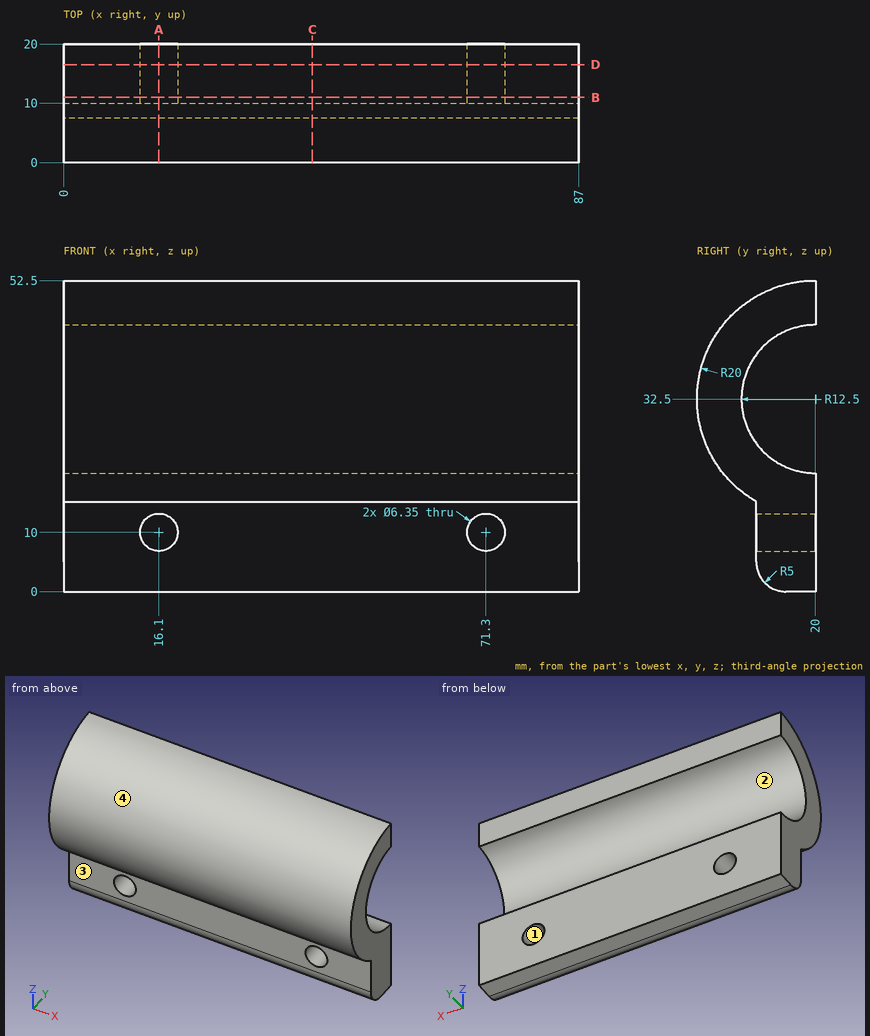
Here's the drawing with two shaded views (mm, measured from the low corner). I have some questions. Coordinates: 2 decimals unless noted, no trailing zeros. Loops run counter-clockwise (first coordinate to the right, second up) from the corner with the lowest first, then second, coordinate; pieces in that order, holes last. Notation, with made-up numbers: (24, 89.25) -> (69, 89.25) arc R24 ccw to (69, 111.25) -> close; hole circle Ø10 at (65.5, -38.5). An arc over 180 degrees is marked (long way). Answer in a Markdown table with one row per item.
(1) Imagine slicing it at A-A (x = 16.1). List the corners of the cut face in (y, z) for me (1 decimal), plus the area to 3 significant figures.
Results found:
| item | result |
|---|---|
| outline | (10, 5) arc R5 ccw to (15, 0) -> (20, 0) -> (20, 6.8) -> (10, 6.8) -> close; (10, 13.2) -> (20, 13.2) -> (20, 20) arc R12.5 cw to (20, 45) -> (20, 52.5) arc R20 ccw to (10, 15.2) -> close |
| area | 448 mm^2 |
(2) Imagine slicing it at B-B (y = 11). List the corners of the cut face in (x, z) for me (3 decimals), plus the area to 3 significant figures.
Results found:
| item | result |
|---|---|
| outline | (0, 2) -> (87, 2) -> (87, 23.825) -> (0, 23.825) -> close; (0, 41.175) -> (87, 41.175) -> (87, 50.361) -> (0, 50.361) -> close; hole circle Ø6.35 at (16.1, 10); hole circle Ø6.35 at (71.3, 10) |
| area | 2,630 mm^2 |
(3) Thinking about a two-plate mould opening in Z: for the marked faces 1, 2, 3 and 4, which applies, released by +Z, released by -Z, zero draft, split by the parting line, or undercut?
Results found:
| item | result |
|---|---|
| face 1 | undercut |
| face 2 | undercut |
| face 3 | zero draft |
| face 4 | split by the parting line |
(4) Will these pins go through, and if not, where does the flat tip stop? pin 1 Ø7.5 at (x, z) = (71.3, 10) entering from -Y; pin 2 Ø5.5 at (x, z) = (16.1, 10) entering from -Y; pin 3 Ø8 at (x, y) = (73, 6.5) entering from +Z; pin 4 Ø6 at (x, y) = (21, 14) entering from +Z.
Results found:
| item | result |
|---|---|
| pin 1 | stops at y = 10 |
| pin 2 | passes through |
| pin 3 | stops at z = 50.1 |
| pin 4 | stops at z = 52.27 |
(5) Imagine slicing it at D-D (y = 16.5). List the corners of the cut face in (x, z) for me (3 decimals), plus the area to 3 significant figures.
Results found:
| item | result |
|---|---|
| outline | (0, 0) -> (87, 0) -> (87, 20.5) -> (0, 20.5) -> close; (0, 44.5) -> (87, 44.5) -> (87, 52.191) -> (0, 52.191) -> close; hole circle Ø6.35 at (16.1, 10); hole circle Ø6.35 at (71.3, 10) |
| area | 2,390 mm^2 |
(6) Imagine slicing it at C-C (x = 42). List the corners of the cut face in (y, z) for me.
Results found:
| item | result |
|---|---|
| outline | (10, 5) arc R5 ccw to (15, 0) -> (20, 0) -> (20, 20) arc R12.5 cw to (20, 45) -> (20, 52.5) arc R20 ccw to (10, 15.18) -> close |
(7) If I drill on probe 1 along X at (y, z) = (16.5, 10) (3 decimals); probe 2 along Z at (x, y) = (16.1, 15.75) (3 decimals); probe 3 along Z at (x, y) = (16.1, 13.75) (3 decimals), over which ranges is the centre line in solid material (lowest first)?
Results found:
| item | result |
|---|---|
| probe 1 | x = 0 to 12.925, 19.275 to 68.125, 74.475 to 87 |
| probe 2 | z = 0 to 6.825, 13.175 to 20.745, 44.255 to 52.043 |
| probe 3 | z = 0.159 to 6.825, 13.175 to 21.675, 43.325 to 51.498 |
